Part model, mm, in its own coordinate system. A direction names the side the tool comes from. Give positions to 0.01 mm unless a question says otherwise; leave off trailing zeros. Order: outer loops, then holes, each group sorted by start corner. A loop starts at its lowest first (then second) coordinate and runs counter-clockwise, first axis right, second up.
Autodesk Inventor part; units mm, degrees
ref_plane "YZ Plane" through (0, 0, 0) normal (1, 0, 0) x (0, 1, 0)
ref_plane "XZ Plane" through (0, 0, 0) normal (0, 1, 0) x (-1, 0, 0)
ref_plane "XY Plane" through (0, 0, 0) normal (0, 0, 1) x (1, 0, 0)
sketch "Sketch1" plane through (0, 0, 0) normal (0, 0, 1) x (1, 0, 0)
  line L0 (12.7, -50.8) -> (-12.7, -50.8)
  line L1 (-12.7, -50.8) -> (-12.7, 50.8)
  line L2 (-12.7, 50.8) -> (12.7, 50.8)
  line L3 (12.7, 50.8) -> (12.7, -50.8)
  line L4 (12.7, -50.8) -> (-12.7, 50.8) construction
  line L5 (-12.7, -50.8) -> (12.7, 50.8) construction
  point P0 (0, 0)
  dimension "d0" = 25.4
  dimension "d1" = 101.6
extrude "Plate1" add sketch "Sketch1" along normal blind 0.889
sketch "Sketch2" plane through (12.7, 49.911, 0.889) normal (0, 1, 0) x (-1, 0, 0)
  line L0 (25.4, 0) -> (0, 0)
  line L1 (0, 0) -> (0, -76.2)
  line L2 (0, -76.2) -> (25.4, -76.2)
  line L3 (25.4, -76.2) -> (25.4, 0)
edge flange "Flange1" height 76.2 angle 90 thickness 0.889 bend radius 0.889 thickness toward (0, 1, 0) relief straight relief width 0.889 relief depth 0.4445 corner gap 0.889 corner form 0 edges at (0, 50.8, 0) (0, -50.8, 0) wall of the first edge with corners at (-12.7, 49.911, 0.889) (12.7, 49.911, 0.889) (12.7, 49.911, -75.311) (-12.7, 49.911, -75.311)
bend "Bend1"
corner "Corner1"
sketch "Sketch3" plane through (-12.7, 49.911, -74.422) normal (0, 0, -1) x (-1, 0, 0)
  line L0 (-25.4, 0) -> (0, 0)
  line L1 (0, 0) -> (0, 12.7)
  line L2 (0, 12.7) -> (-25.4, 12.7)
  line L3 (-25.4, 12.7) -> (-25.4, 0)
edge flange "Flange2" height 12.7 angle 90 thickness 0.889 bend radius 0.889 thickness toward (0, 0, -1) relief straight relief width 0.889 relief depth 0.4445 corner gap 0.889 corner form 0 edges at (0, 50.8, -75.311) (0, -50.8, -75.311) wall of the first edge with corners at (12.7, 49.911, -74.422) (-12.7, 49.911, -74.422) (-12.7, 62.611, -74.422) (12.7, 62.611, -74.422)
bend "Bend2"
corner "Corner2"
fillet "Corner Round1" radius 6.35 4 edges at (-12.7, 62.611, -74.8665) (12.7, 62.611, -74.8665) (-12.7, -62.611, -74.8665) (12.7, -62.611, -74.8665)
equation "\"d2\" = Thickness"
equation "\"d3\" = BendReliefWidth"
equation "\"d4\" = BendReliefDepth"
equation "\"d5\" = MinimumRemnant"
equation "\"d6\" = TransitionRadius"
equation "\"d9\" = BendRadius"
equation "\"d10\" = CornerReliefSize"
equation "\"d11\" = GapSize"
equation "\"d12\" = JacobiRadiusSize"
equation "\"d13\" = BendReliefWidth"
equation "\"d14\" = BendReliefDepth"
equation "\"d15\" = MinimumRemnant"
equation "\"d16\" = TransitionRadius"
equation "\"d19\" = BendRadius"
equation "\"d20\" = CornerReliefSize"
equation "\"d21\" = GapSize"
equation "\"d22\" = JacobiRadiusSize"
equation "\"BendRadius\" = Thickness"
equation "\"BendReliefWidth\" = Thickness"
equation "\"BendReliefDepth\" = 0.5 * Thickness"
equation "\"CornerReliefSize\" = 4 * Thickness"
equation "\"MinimumRemnant\" = 2 * Thickness"
equation "\"TransitionRadius\" = BendRadius"
equation "\"JacobiRadiusSize\" = Thickness"
equation "\"GapSize\" = Thickness"
properties part number "Handle" material "Aluminum 6061"
Item 1: Band-saw the part on D-D on x = -8. List the corners of the cut face in (y, z), plus the area to 3 significant figures.
Item 2: Drill centre lines: probe 1 along Y at (x, z) = (2.5, -24.5); probe 2 along Z at (x, y) = (-3.75, -23); probe 3 along Z at (x, y) = (-5, 56.5). Where is each one in solid material? Low to high.
Item 3: Drop flat-ended pins along their axis: P1, Ø5.5, axis at x = -0.5, y = -59, coming from the +Z side; P2, Ø6, axis at x = -8.5, y = 13, coming from the -Z side; P3, Ø4, axis at x = -3, z = -32, coming from the -Y side; P4, Ø6, axis at x = -2.5, y = -49.5, coming from the +Z side. Give the stop position or say it passes through.
Item 4: Band-saw the part on B-B on x = -0.5. List the corners of the cut face in (y, z).
Item 5: Band-saw the part on A-A on z = -25.5. List the corners of the cut face in (x, y).
Item 6: Band-saw the part on C-C on y = 47.5. List the corners of the cut face in (x, z).
Item 7: Pull direction Y, two halves, no side cores. Call faces 6 (the face through (-10.89, 60.7, -74.87)), 7 (the face through (0, 1, 0)), 8 (the face through (0, 57, -75.311)): released by +Y, released by -Y, zero draft, split by the parting line, or undercut.
Item 8: Which spindle directions (+Z, -Z, +X, -X, +Y, -Y) get a long thin tool onto all of the face, cutting with end or side? Do faces 1 (the face through (-12.7, 50.3, -37.4)), 2 (the face through (0, -57, -74.422)), 3 (the face through (0, 1, 0.889)), 4 (the face through (0, 50.8, -38)), 5 (the face through (0, 49.911, -37)). Say none if no direction does.
Working result:
1. outline: (-62.39, -75.31) - (-51.69, -75.31) arc R1.78 ccw to (-49.91, -73.53) - (-49.91, -0.89) arc R0.89 cw to (-49.02, 0) - (49.02, 0) arc R0.89 cw to (49.91, -0.89) - (49.91, -73.53) arc R1.78 ccw to (51.69, -75.31) - (62.39, -75.31) - (62.39, -74.42) - (51.69, -74.42) arc R0.89 cw to (50.8, -73.53) - (50.8, -0.89) arc R1.78 ccw to (49.02, 0.89) - (-49.02, 0.89) arc R1.78 ccw to (-50.8, -0.89) - (-50.8, -73.53) arc R0.89 cw to (-51.69, -74.42) - (-62.39, -74.42) - close
1. area: 243 mm2
2. probe 1: y = -50.8 to -49.91, 49.91 to 50.8
2. probe 2: z = 0 to 0.89
2. probe 3: z = -75.31 to -74.42
3. P1: stops at z = -74.42
3. P2: stops at z = 0
3. P3: stops at y = -50.8
3. P4: stops at z = 0.89
4. outline: (-62.61, -75.31) - (-51.69, -75.31) arc R1.78 ccw to (-49.91, -73.53) - (-49.91, -0.89) arc R0.89 cw to (-49.02, 0) - (49.02, 0) arc R0.89 cw to (49.91, -0.89) - (49.91, -73.53) arc R1.78 ccw to (51.69, -75.31) - (62.61, -75.31) - (62.61, -74.42) - (51.69, -74.42) arc R0.89 cw to (50.8, -73.53) - (50.8, -0.89) arc R1.78 ccw to (49.02, 0.89) - (-49.02, 0.89) arc R1.78 ccw to (-50.8, -0.89) - (-50.8, -73.53) arc R0.89 cw to (-51.69, -74.42) - (-62.61, -74.42) - close
5. outline: (-12.7, -50.8) - (12.7, -50.8) - (12.7, -49.91) - (-12.7, -49.91) - close; (-12.7, 49.91) - (12.7, 49.91) - (12.7, 50.8) - (-12.7, 50.8) - close
6. outline: (-12.7, 0) - (12.7, 0) - (12.7, 0.89) - (-12.7, 0.89) - close
7. face 6: released by +Y
7. face 7: undercut
7. face 8: zero draft
8. face 1: +Z, -Z, -X, +Y, -Y
8. face 2: +Z, +X, -X, -Y
8. face 3: +Z, +X, -X, +Y, -Y
8. face 4: +Z, +X, -X, +Y
8. face 5: -Z, +X, -X
